The listing builds one solid part. Answer for the finished solid, in the listing's coordinates (mm). A direction names the side the tool comes from. Give positions to 0.01 mm unless a question says otherwise; leave off trailing zeros. Write each loop counter-clockwise with the first axis right and the second up, starting at its lowest first coordinate (ties: lowest second). Pieces come first, ordered by that corner, then holes. Notation, with made-up numbers: M -21.5,34.5 L 19.5,34.5 A24 cw 19.5,50.5 Z; hole C 31,-38 d5. An arc over 180 degrees is marked long. Return JSON: item names as keys, results as strings.
Autodesk Inventor part; units mm, degrees
ref_plane "YZ Plane" through (0, 0, 0) normal (1, 0, 0) x (0, 1, 0)
ref_plane "XZ Plane" through (0, 0, 0) normal (0, 1, 0) x (-1, 0, 0)
ref_plane "XY Plane" through (0, 0, 0) normal (0, 0, 1) x (1, 0, 0)
sketch "Sketch1" plane through (0, 0, 0) normal (0, 1, 0) x (-1, 0, 0)
  line L0 (5.8568, 1.9857) -> (-14.1432, 1.9857)
  line L1 (-14.1432, 1.9857) -> (-14.1432, -5.0143)
  line L2 (-14.1432, -5.0143) -> (5.8568, -5.0143)
  line L3 (5.8568, -5.0143) -> (5.8568, 1.9857)
  line L4 (7.3568, 3.4857) -> (-15.6432, 3.4857)
  line L5 (-15.6432, 3.4857) -> (-15.6432, -6.5143)
  line L6 (-15.6432, -6.5143) -> (7.3568, -6.5143)
  line L7 (7.3568, -6.5143) -> (7.3568, 3.4857)
  line L8 (7.3568, 3.4857) -> (-15.6432, 3.4857)
  line L9 (-15.6432, 3.4857) -> (-15.6432, 6.4857)
  line L10 (-15.6432, 6.4857) -> (7.3568, 6.4857)
  line L11 (7.3568, 6.4857) -> (7.3568, 3.4857)
  line L12 (7.3568, -6.5143) -> (-15.6432, -6.5143)
  line L13 (-15.6432, -6.5143) -> (-15.6432, -9.5143)
  line L14 (-15.6432, -9.5143) -> (7.3568, -9.5143)
  line L15 (7.3568, -9.5143) -> (7.3568, -6.5143)
  point P0 (0, 0)
  dimension "d0" = 20
  dimension "d1" = 7
  dimension "d2" = 1.5
  dimension "d3" = 3
  dimension "d4" = 3
extrude "Extrusion1" add sketch "Sketch1" along normal blind 0.6 contours L7 L6 L5 L4
extrude "Extrusion2" add sketch "Sketch1" along normal blind 7.6 contours L4 L9 L10 L11 | L15 L14 L13 L6
fillet "Fillet1" radius 2 4 edges at (-7.3568, 7.6, 4.9857) (15.6432, 7.6, -8.0143) (15.6432, 7.6, 4.9857) (-7.3568, 7.6, -8.0143)
sketch "Sketch2" plane through (0, 0.6, 0) normal (0, 1, 0) x (1, 0, 0)
  line L0 (-8.4877, 1.4143) -> (-3.1279, 1.4143)
  line L1 (-3.1279, 1.4143) -> (-3.1279, 1.6143)
  line L2 (-3.1279, 1.6143) -> (-8.4877, 1.6143)
  line L3 (-8.4877, 1.6143) -> (-8.4877, 1.4143)
  line L4 (-5.8568, -1.9857) -> (-5.8568, 5.0143)
  point P0 (0, 0)
  point P1 (-5.8568, 1.5143)
  point P2 (-8.4877, 1.5143)
  dimension "d10" = 0.2
extrude "Extrusion3" cut sketch "Sketch2" against normal through all
properties part number "oslona_wlacznika"
Item 1: A cutting plane is placed at A-A, the plane z = -4.25. Write down the section's boundary in (x, y).
Geometry results:
{"outline": "M -7.36,0 L -5.86,0 L -5.86,0.6 L -7.36,0.6 Z; M 14.14,0 L 15.64,0 L 15.64,0.6 L 14.14,0.6 Z"}
Item 2: Which of the six approach directions +Z, -Z, +X, -X, +Y, -Y give full straight-line access (tool end or side, diameter ignored) to faces 5 (the flat face through (4, 4, -6.514)), 6 (the flat face through (4, 7.6, 5))?
Geometry results:
{"face 5": "+X, -X, +Y", "face 6": "+Z, -Z, +X, -X, +Y"}
Item 3: Determine the mould class of faces 1 (the flat face through (4.3, 0, 2.2)), 2 (the flat face through (4, 0.6, -6)), 3 (the flat face through (4, 4, 6.486)), 4 (the flat face through (4, 4, 3.486)) for opening direction Z: +Z half, -Z half, draft (parallel to the pull), parting line (faces both ways), or undercut.
Geometry results:
{"face 1": "draft", "face 2": "undercut", "face 3": "+Z half", "face 4": "undercut"}
Item 4: A cutting plane is placed at C-C, the plane x = 7.75. Write down the section's boundary in (y, z).
Geometry results:
{"outline": "M 0,-9.51 L 7.6,-9.51 L 7.6,-6.51 L 0.6,-6.51 L 0.6,-5.01 L 0,-5.01 Z; M 0,1.99 L 0.6,1.99 L 0.6,3.49 L 7.6,3.49 L 7.6,6.49 L 0,6.49 Z"}
Item 5: Find the intervals of material crossed by line 1 (Z direction, x = 7, y = 3); line 2 (Y direction, x = 4.75, z = 3.25); line 3 (X direction, y = 6.5, z = 4.5), in increasing order.
Geometry results:
{"line 1": "z = -9.51 to -6.51, 3.49 to 6.49", "line 2": "y = 0 to 0.6", "line 3": "x = -7.14 to 15.43"}
Item 6: A cutting plane is placed at B-B, the plane y = 3.5. Write down the section's boundary in (x, z).
Geometry results:
{"outline": "M -7.36,-9.51 L 15.64,-9.51 L 15.64,-6.51 L -7.36,-6.51 Z; M -7.36,3.49 L 15.64,3.49 L 15.64,6.49 L -7.36,6.49 Z"}
Item 7: Given pin 1 Ø5 at (x, z) = (9, -1) entering from +Y; pin 2 Ø5 at (x, z) = (-2.5, 1) entering from -Y, each flat-ended and moving along its own axis, determine where each tip first touches the part or whether it passes through.
Geometry results:
{"pin 1": "passes through", "pin 2": "stops at y = 0"}
